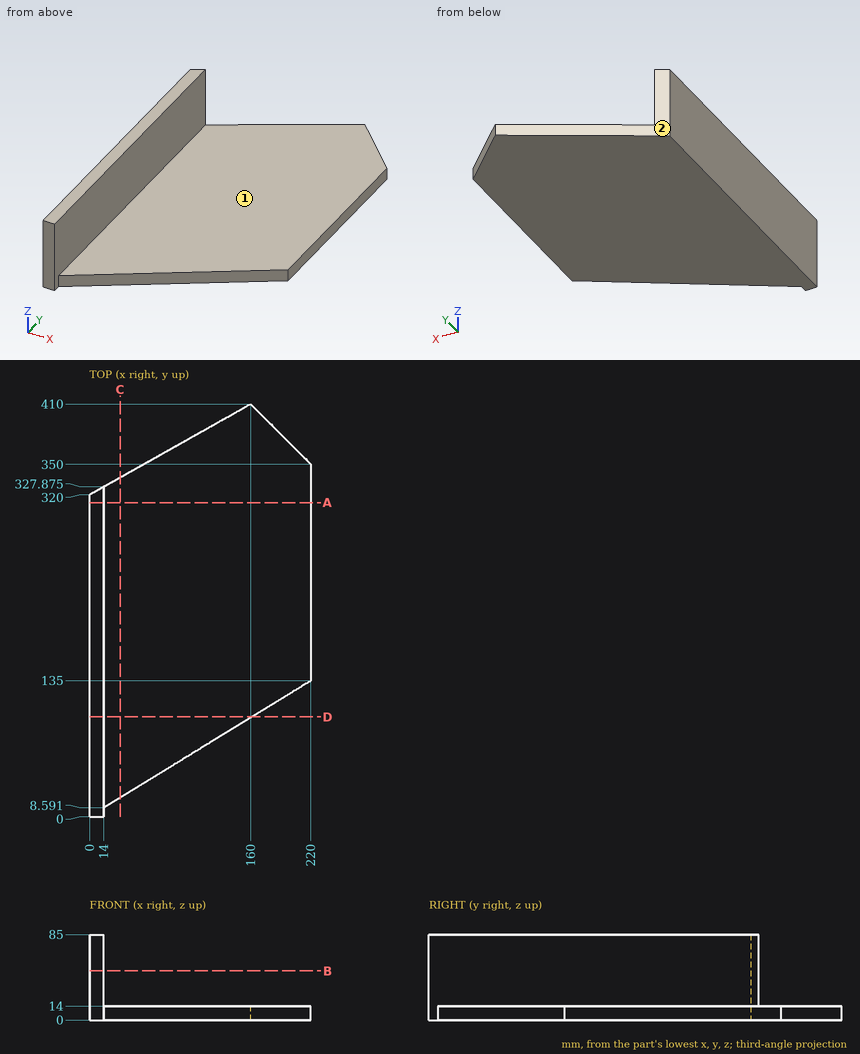
Input: dimensioned drawing with shaded views. Units: mm. Origin: part minimum x, y, z. A direction names the side the tool comes from. Give positions to 0.01 mm unless a question says otherwise; leave off trailing zeros. Write each loop counter-clockwise with the first axis right and the second up, starting at its lowest first coordinate (ties: lowest second). Pieces come first, ordered by that corner, then holes. Notation, with made-up numbers: (22, -31) -> (76, -31) arc R34 ccw to (76, 8) -> close; hole circle Ø11 at (51, 17.25). An arc over 180 degrees is marked (long way). Answer as a JSON object with one key per item and string values.
1. Contact query for flat-ended pins moving along their axis: pin 1 (10 mm diameter, centred on y = 231, z = 60.5, fed in from -X); pin 2 (4 mm diameter, centred on x = 133.5, y = 268, fed in from +Z). Output: stop coordinate, or through.
Ans:
{"pin 1": "stops at x = 0", "pin 2": "stops at z = 14"}
2. Cut plane C-C on x = 30.5. Output: boundary loops of the cut face in (y, z).
Ans:
{"outline": "(18.72, 0) -> (337.16, 0) -> (337.16, 14) -> (18.72, 14) -> close"}
3. Cut plane D-D on y = 99. Output: boundary loops of the cut face in (x, z), and give its area (3 significant figures).
Ans:
{"outline": "(0, 0) -> (161.33, 0) -> (161.33, 14) -> (14, 14) -> (14, 85) -> (0, 85) -> close", "area": "3,250 mm^2"}
4. Ray query, probe 1 along Z at (x, y) = (42.5, 76); probe 2 along Y at (x, z) = (118, 4) (1 decimal). Return the intervals inside material, ascending. Write a range as from..to.
Ans:
{"probe 1": "z = 0..14", "probe 2": "y = 72.4..386.4"}
5. Cut plane B-B on z = 49. Output: boundary loops of the cut face in (x, y) (3 decimals).
Ans:
{"outline": "(0, 0) -> (14, 0) -> (14, 327.875) -> (0, 320) -> close"}
6. Cut plane A-A on y = 312. Output: boundary loops of the cut face in (x, z).
Ans:
{"outline": "(0, 0) -> (220, 0) -> (220, 14) -> (14, 14) -> (14, 85) -> (0, 85) -> close"}
7. Access query for the marked faces 1 and 2. Directions: +Z, -Z, +X, -X, +Y, -Y. A direction counts if a zero-diameter tool reaches every point of the face in a straight line with its end or side. Return the directions, or none.
Ans:
{"face 1": "+Z, +X, +Y, -Y", "face 2": "+Z, -Z, -X, +Y"}
